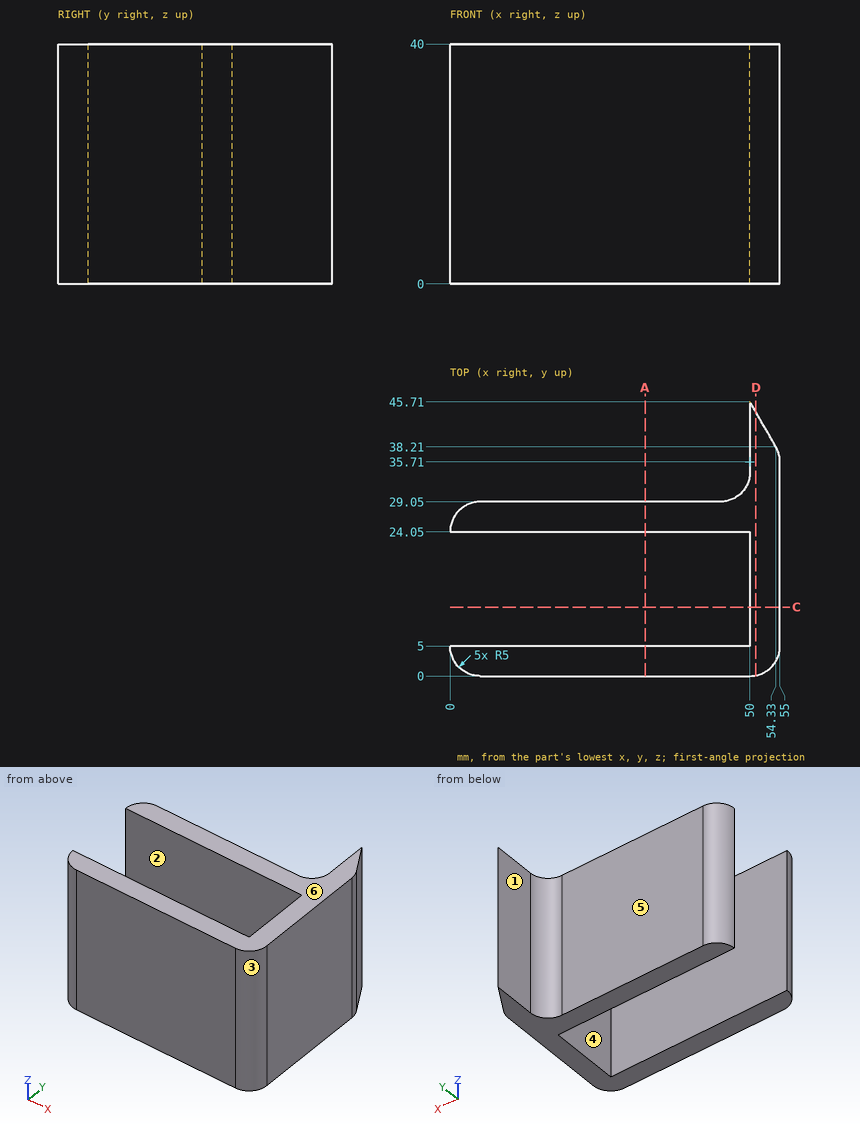
Verification items for this drawing (mm, ordinates from the low corner). A direction names the side the tool comes from. Coordinates: 2 decimals unless noted, no trailing zeros. Order: outer loops, then holes, each group sorted by start corner. A loop starts at its lowest first (then second) coordinate and runs counter-clockwise, first axis right, second up. Notation, with made-up numbers: (-23.5, -37) -> (1.5, -37) arc R17 ccw to (1.5, -27) -> close; hole circle Ø4 at (65, 6.25). An arc over 180 degrees is marked (long way). Put each result on its own line as item: value. Start each with the question number.
1. Cross-section at A-A, the plane x = 32.5. Record the boundary of the cut face in (y, z), then the cut area to 3 significant figures.
2. Cross-section at C-C, the plane y = 11.5. Record the boundary of the cut face in (x, z).
3. Go/stop test with flat-tipped pins: pin 1 Ø3 at (y, z) = (41, 16) entering from -X; pin 2 Ø6 at (y, z) = (39.5, 11) entering from +X; pin 3 Ø12 at (x, z) = (25.5, 15) entering from +Y. Record where each tip stops, or that it passes through.
4. Cross-section at D-D, the plane x = 51. Record the boundary of the cut face in (y, z), then the cut area to 4 significant figures.
5. Material ranges on L1, parallel to Y at x = 42.5, z = 28.5; L2, parallel to X at y = 19, z = 16, recorded low to high. Write a range as [from, to].
6. Access from +Z, -Z, +X, -X, +Y, -Y to the whole of each face (thin tool, end or side, straight path). Record for the marked faces 1, 2 and 3.
7. Mould release check, pull along Y, two halves, no side actions. Record for the marked faces 4, 5 and 6: released by +Y, released by -Y, zero draft, split by the parting line, or undercut.
Computed:
1. outline: (0, 0) -> (5, 0) -> (5, 40) -> (0, 40) -> close; (24.05, 0) -> (29.05, 0) -> (29.05, 40) -> (24.05, 40) -> close
1. area: 400 mm2
2. outline: (50, 0) -> (55, 0) -> (55, 40) -> (50, 40) -> close
3. pin 1: x = 50
3. pin 2: x = 54.94
3. pin 3: y = 29.05
4. outline: (0.1, 0) -> (43.98, 0) -> (43.98, 40) -> (0.1, 40) -> close
4. area: 1,755 mm2
5. L1: [0, 5], [24.05, 29.05]
5. L2: [50, 55]
6. face 1: +Z, -Z, -X, +Y
6. face 2: +Z, -Z, -X
6. face 3: +Z, -Z, +X, -Y
7. face 4: undercut
7. face 5: released by +Y
7. face 6: zero draft
